```python
from build123d import *

# Parameters (mm, degrees)
SKETCH1_R           = 2.1
BOSS_EXTRUDE1_DEPTH = 161.5


with BuildPart() as part:
    # Sketch1 → Boss-Extrude1 (new body)
    with BuildSketch(Plane.XY):
        Polygon((-10, 10), (-4.25, 10), (-3.065, 8.2), (-5.5, 8.2), (-5.5, 6.348528137), (-3.051471863, 3.9), (0, 3.9), (3.051471863, 3.9), (5.5, 6.348528137), (5.5, 8.2), (3.065, 8.2), (4.25, 10), (10, 10), (10, 4.25), (8.2, 3.065), (8.2, 5.5), (6.348528137, 5.5), (3.9, 3.051471863), (3.9, 0), (3.9, -3.051471863), (6.348528137, -5.5), (8.2, -5.5), (8.2, -3.065), (10, -4.25), (10, -10), (4.25, -10), (3.065, -8.2), (5.5, -8.2), (5.5, -6.348528137), (3.051471863, -3.9), (0, -3.9), (-3.051471863, -3.9), (-5.5, -6.348528137), (-5.5, -8.2), (-3.065, -8.2), (-4.25, -10), (-10, -10), (-10, -4.25), (-8.2, -3.065), (-8.2, -5.5), (-6.348528137, -5.5), (-3.9, -3.051471863), (-3.9, 0), (-3.9, 3.051471863), (-6.348528137, 5.5), (-8.2, 5.5), (-8.2, 3.065), (-10, 4.25), align=None)
        Circle(SKETCH1_R, mode=Mode.SUBTRACT)
    extrude(amount=BOSS_EXTRUDE1_DEPTH)


solid = part.part
```
Build history of the part. All positions in model axes, mm. A direction names the side the tool comes from. Give positions to 0.01 mm unless a question says otherwise; leave off trailing zeros. Order: outer loops, then holes, each group sorted by start corner. A loop starts at its lowest first (then second) coordinate and runs counter-clockwise, first axis right, second up. Notation, with made-up numbers: M -25.5,67.5 L 25.5,67.5 A26 ccw 25.5,101.5 Z; hole C -31,36 d3. An arc over 180 degrees is marked long. Write item = value, one per line. Start each with the question number.
(1) Probe L1, parallel to Y at x = 0, z = 33; L2, parallel to Y at x = 5, z = 61.5; L3, parallel to Y at x = 4.5, z = 60. List the from-to ranges inside material, lowest first. Write a range as [from, to].
(2) Which spindle directions (+Z, -Z, +X, -X, +Y, -Y) get a long thin tool onto all of the face, cutting with end or side? Do faces 1 (the flat face through (-10, -7, 80)), 2 (the flat face through (3.9, 0, 80)), 3 (the flat face through (7, -10, 80)), 4 (the flat face through (0, 3.9, 80)), 5 (the flat face through (0, -3.9, 80)). Say none if no direction does.
(3) Pin check, flat tips, straight feed: pin 1 Ø4 at (y, z) = (1.5, 88) entering from +X; pin 2 Ø1 at (y, z) = (-3.5, 22) entering from +X; pin 3 Ø3 at (x, z) = (0.5, 82.5) entering from -Y. Stop position of each tip, or through.
(4) Slice it at A-A on y = 0. Write the cut outline in (x, z).
(5) Two-plate mould, pull along Y, no slides. Class faces 6 (the flat face through (0.1, 2.4, 161.5)), 7 (the flat face through (-3.9, 0, 80)), 8 (the cylindrical face through (2.003, 0.631, 79.62)), 9 (the flat face through (7, 10, 80)): released by +Y, released by -Y, zero draft, split by the parting line, or undercut.
Responses:
q1.L1 = [-3.9, -2.1], [2.1, 3.9]
q1.L2 = [-10, -8.2], [-5.85, -4.15], [4.15, 5.85], [8.2, 10]
q1.L3 = [-10, -8.2], [-5.35, -3.65], [3.65, 5.35], [8.2, 10]
q2.face_1 = +Z, -Z, -X, +Y, -Y
q2.face_2 = +Z, -Z, +X
q2.face_3 = +Z, -Z, +X, -X, -Y
q2.face_4 = +Z, -Z, +Y
q2.face_5 = +Z, -Z, -Y
q3.pin_1 = 8.86
q3.pin_2 = 9.62
q3.pin_3 = -3.9
q4.outline = M -3.9,0 L -2.1,0 L -2.1,161.5 L -3.9,161.5 Z; M 2.1,0 L 3.9,0 L 3.9,161.5 L 2.1,161.5 Z
q5.face_6 = zero draft
q5.face_7 = undercut
q5.face_8 = undercut
q5.face_9 = released by +Y
